For this review, use the dimensioned drawing (mm, ordinates from the lowest corner) and the shaded views. Round coordinates to 2 decimals unless told otherwise and drop trailing zeros. Loops run counter-clockwise (first coordinate to the right, second up) from the corner with the lowest first, then second, coordinate; pieces in that order, holes last. Notation, with made-up numbers: (6, 13.5) - (60, 13.5) arc R36 cw to (60, 47.5) - close; hole circle Ø8 at (58, -23.75). An arc over 180 degrees is marked (long way). Answer as CSV lines item,"result". Start each with the question number.
(1) Consider section D-D (z = 15.5). Give the boundary of the cut face in (x, y), and give its area (3 significant figures).
(2) Consider section C-C (y = 5.5). Give the boundary of the cut face in (x, z), and give its area (3 significant figures).
(3) Consider section A-A (z = 20). Give the boundary of the cut face in (x, y).
(4) Wall thickness on L1, parallel to X at y = 12.5, z = 20; L2, parallel to Y at x = 8.5, z = 32.5; L3, parallel to Z at x = 20.5, y = 1.75: over which ranges is each line inside the solid? List them lowest first.
(5) For P1, Ø5, axis at x = 20, z = 20, coming from the -Y side; P2, Ø6, axis at x = 23.5, y = 3.5, coming from the +Z side; P3, Ø5, axis at y = 12, z = 26.5, coming from the -X side; P4, Ø4, axis at y = 13.5, z = 16, coming from the -X side, all flat-tipped, find the tip position at first contact; note any pin that passes through.
(6) Mouldability with a two-part tool opening along X and no side actions: class the marked faces 1, 2 and 3 as released by +X, released by -X, zero draft, split by the parting line, or undercut.
(7) Consider section B-B (x = 20). Give the boundary of the cut face in (y, z), and give its area (3 significant figures).
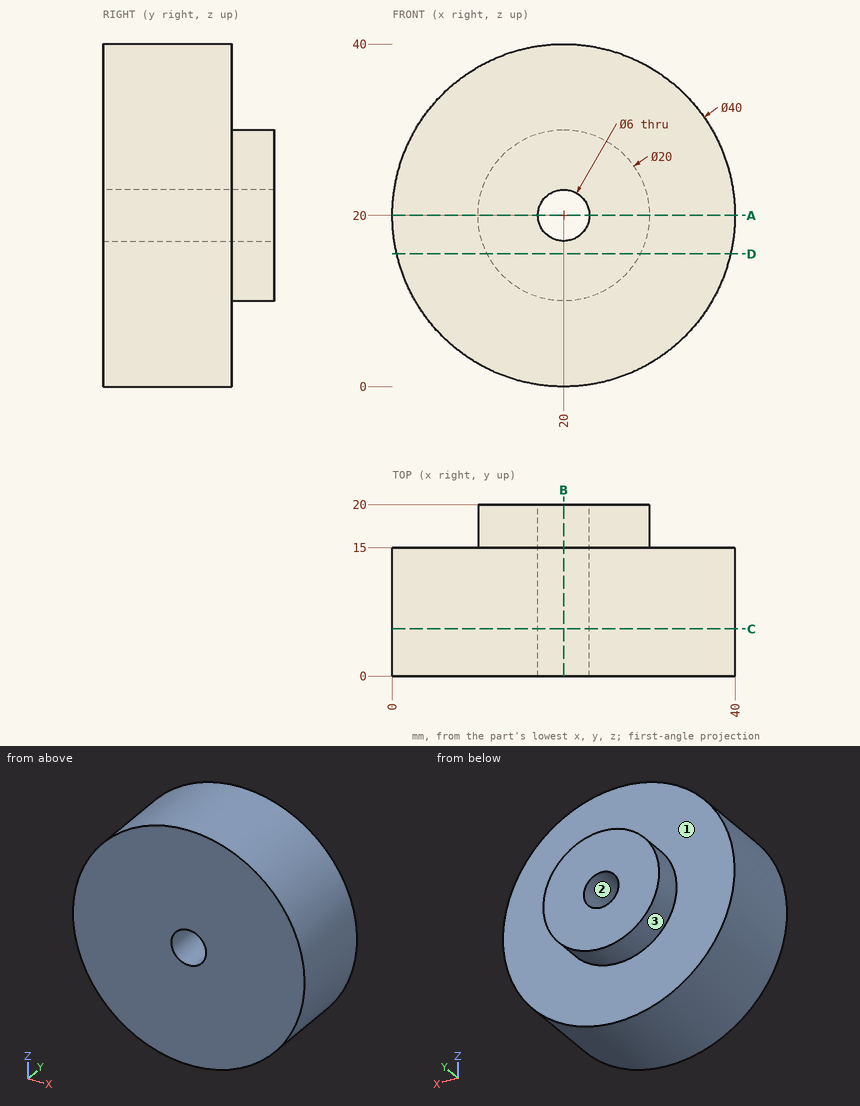
Determined:
1,outline,"(0.51, 0) - (39.49, 0) - (39.49, 15) - (28.93, 15) - (28.93, 20) - (11.07, 20) - (11.07, 15) - (0.51, 15) - close"
1,area,"674 mm^2"
2,outline,"circle Ø40 at (20, 20); hole circle Ø6 at (20, 20)"
2,area,"1,230 mm^2"
3,outline,"(0, 0) - (17, 0) - (17, 20) - (10, 20) - (10, 15) - (0, 15) - close; (23, 0) - (40, 0) - (40, 15) - (30, 15) - (30, 20) - (23, 20) - close"
4,L1,"x = 0 to 17, 23 to 40"
4,L2,"y = 0 to 15"
4,L3,"z = 0.01 to 17.04, 22.96 to 39.99"
5,P1,"passes through"
5,P2,"stops at z = 39.99"
5,P3,"stops at x = 0.4"
5,P4,"stops at x = 0.1"
6,face 1,"zero draft"
6,face 2,"undercut"
6,face 3,"split by the parting line"
7,outline,"(0, 0) - (15, 0) - (15, 10) - (20, 10) - (20, 17) - (0, 17) - close; (0, 23) - (20, 23) - (20, 30) - (15, 30) - (15, 40) - (0, 40) - close"
7,area,"580 mm^2"
